```python
from build123d import *

# Parameters (mm, degrees)
SKETCH1_R           = 12.95
BOSS_EXTRUDE1_DEPTH = 3.175
CHAMFER1_SIZE       = 0.4


with BuildPart() as part:
    # Sketch1 → Boss-Extrude1 (new body)
    with BuildSketch(Plane(origin=(0, 0, 0), x_dir=(1, 0, 0), z_dir=(0, 1, 0))):
        with Locations(Location((0, 0, 0), (0, 0, 270))):
            Circle(SKETCH1_R)
        Polygon((0.60374079, 7.597071611), (-6.277386614, 4.321390667), (-6.881127404, -3.275680944), (-0.60374079, -7.597071611), (6.277386614, -4.321390667), (6.881127404, 3.275680944), align=None, mode=Mode.SUBTRACT)
    extrude(amount=BOSS_EXTRUDE1_DEPTH)

    # Chamfer1
    chamfer1_edges = [part.edges().sort_by_distance(p)[0] for p in [
        (-6.579257009, 0, -0.522854862),
        (-3.742434097, 0, 5.436376277),
        (2.836822912, 0, 5.959231139),
        (6.579257009, 0, 0.522854862),
        (0, 0, -12.95),
        (3.742434097, 0, -5.436376277),
        (-2.836822912, 0, -5.959231139),
    ]]
    chamfer(chamfer1_edges, length=CHAMFER1_SIZE)


solid = part.part
```
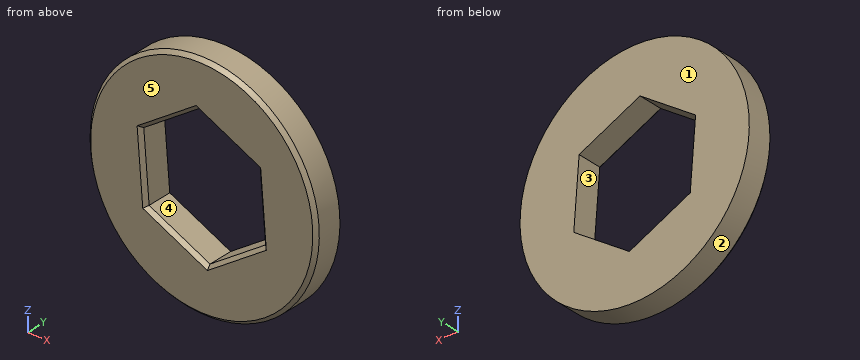
Could you check a few things on this model? Use its own coordinates, in mm. Face numbers are marked on the shaded views. A direction names the side the tool comes from. Round coordinates to 2 decimals unless told otherwise and drop trailing zeros. Write each loop counter-clockwise with the first axis right and the second up, starting at its lowest first coordinate (ties: lowest second). Pieces come first, ordered by that corner, then holes.
(1) Suppose I cut it at A-A on y = 1.15. Write out the boundary of the cut face in (x, z), and give its area (3 significant figures).
Findings below:
outline: circle Ø25.9 at (0, 0); hole (-6.88, 3.28) - (-6.28, -4.32) - (0.6, -7.6) - (6.88, -3.28) - (6.28, 4.32) - (-0.6, 7.6) - close
area: 376 mm2
(2) Suppose I cut it at B-B on x = 0. Write out the boundary of the cut face in (y, z) (3 decimals).
Findings below:
outline: (0, -12.55) - (0.4, -12.95) - (3.175, -12.95) - (3.175, -7.31) - (0.4, -7.31) - (0, -7.753) - close; (0, 7.753) - (0.4, 7.31) - (3.175, 7.31) - (3.175, 12.95) - (0.4, 12.95) - (0, 12.55) - close
(3) For pin 1 (1.5 mm diameter, centred on y = 1, z = 4.5, fed in from +X); pin 2 (1 mm diameter, centred on y = 2, z = 1, fed in from -X), each with a flat end and sliding along its axis, tell me the tip position at first contact or that it passes through.
Findings below:
pin 1: stops at x = 12.4
pin 2: stops at x = -12.94
(4) Which directions (+Z, -Z, +X, -X, +Y, -Y) give clear straight access to the entire face, cutting with the end or side of a thin tool? Please do the marked faces 4 and 5.
Findings below:
face 4: +Y, -Y
face 5: +Z, -Z, +X, -X, -Y
(5) Suppose I cut it at C-C on z = 0. Write out the boundary of the cut face in (x, y) (3 decimals).
Findings below:
outline: (-12.95, 0.4) - (-12.55, 0) - (-7.022, 0) - (-6.621, 0.4) - (-6.621, 3.175) - (-12.95, 3.175) - close; (6.621, 0.4) - (7.022, 0) - (12.55, 0) - (12.95, 0.4) - (12.95, 3.175) - (6.621, 3.175) - close
(6) If I drill on probe 1 along Z at (x, y) = (3.5, 0.3); probe 2 along X at (y, z) = (0.5, -3.5); probe 3 along Z at (x, y) = (-5.5, 2.6), over which ranges is the centre line in solid material (lowest first)?
Findings below:
probe 1: z = -12.36 to -5.72, 5.75 to 12.36
probe 2: x = -12.47 to -6.34, 6.56 to 12.47
probe 3: z = -11.72 to -4.69, 4.23 to 11.72
(7) Thinking about a two-plate mould opening in X: for the marked faces 1, 2 and 3, which applies, +X half, -X half, draft (parallel to the pull), parting line (faces both ways), or undercut?
Findings below:
face 1: draft
face 2: parting line
face 3: undercut
